Geometry check sheet. Reference: drawing and pictorial views, mm from the part's lowest x, y, z. A direction names the side the tool comes from. Give positions to 0.01 mm unless a question says otherwise; leave off trailing zeros. Loops run counter-clockwise (first coordinate to the right, second up) from the corner with the lowest first, then second, coordinate; pieces in that order, holes last. Notation, with made-up numbers: (28, -13.75) -> (77, -13.75) arc R22 cw to (77, 20.25) -> close; hole circle Ø8 at (51, 37). An arc over 180 degrees is marked (long way). One line per item, written item: value. Start each with the question number.
(1) Sectioned sample at B-B, the plane y = 11.75. Record the cut outline in (x, z), then the cut area to 3 significant figures.
(2) Tool access check on the marked faces 4, 5 and 6. Record the directions out of +Z, -Z, +X, -X, +Y, -Y that give a thin tool (end or side, any length) a straight path to the whole face; none if there is none.
(3) Sectioned sample at C-C, the plane z = 15. State how many separate pieces and enclosed holes the cut face has, then the cut area to 3 significant figures.
(4) Scan lines: line 1 along Z through (x, y) = (20, 21.8); line 2 along Y through (x, z) = (88, 13); line 3 along X through (y, z) = (4.5, 24.5). Record each from-to range of solid material in increasing order. Write a range as from..to.
(5) Draft check along Z on the marked faces 1, 2 and 3. Enter one of: pulls with the +Z half, pulls with the -Z half, needs draft (parallel to the pull), parting line crosses it, or undercut.
(6) Sectioned sample at A-A, the plane x = 70. Record the cut outline in (y, z).
(7) Gauge pin test, flat ends, axial feed: pin 1 Ø5 at (x, z) = (80, 23) entering from -Y; pin 2 Ø10 at (y, z) = (10.5, 24.5) entering from -X; pin 3 Ø7.5 at (y, z) = (6.5, 14.5) entering from -X. Record the tip position at first contact, or that the pin passes through.
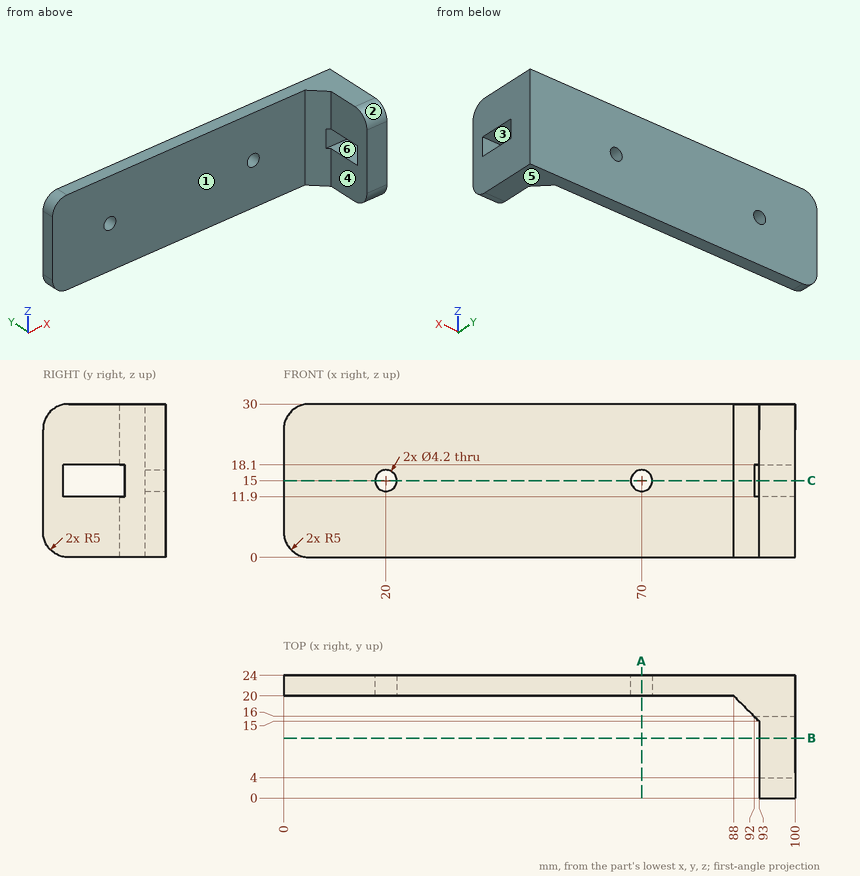
Calculated:
1. outline: (93, 0) -> (100, 0) -> (100, 11.9) -> (93, 11.9) -> close; (93, 18.1) -> (100, 18.1) -> (100, 30) -> (93, 30) -> close
1. area: 167 mm2
2. face 4: +Z, -Z, -X, -Y
2. face 5: -Z, +X, -X, +Y, -Y
2. face 6: +X, -X
3. separate pieces: 4
3. enclosed holes: 0
3. area: 434 mm2
4. line 1: z = 0..12.9, 17.1..30
4. line 2: y = 20..24
4. line 3: x = 93..100
5. face 1: needs draft
5. face 2: pulls with the +Z half
5. face 3: undercut
6. outline: (20, 0) -> (24, 0) -> (24, 12.9) -> (20, 12.9) -> close; (20, 17.1) -> (24, 17.1) -> (24, 30) -> (20, 30) -> close
7. pin 1: stops at y = 20
7. pin 2: stops at x = 92.5
7. pin 3: stops at x = 93
